Can you work these out from the drawing? Everything is in mm from the part's minimum corner. A direction names the side the tool comes from. Round coordinates to 2 decimals unless told otherwise and drop trailing zeros. Order: outer loops, then holes, each group sorted by start corner. A loop starts at its lowest first (then second) coordinate and runs counter-clockwise, first axis right, second up. Notation, with made-up numbers: (41, 75.25) -> (96, 75.25) arc R22 ccw to (96, 95.25) -> close; hole circle Ø11 at (89.25, -3). An arc over 180 degrees is marked (long way). One line per item, written item: value.
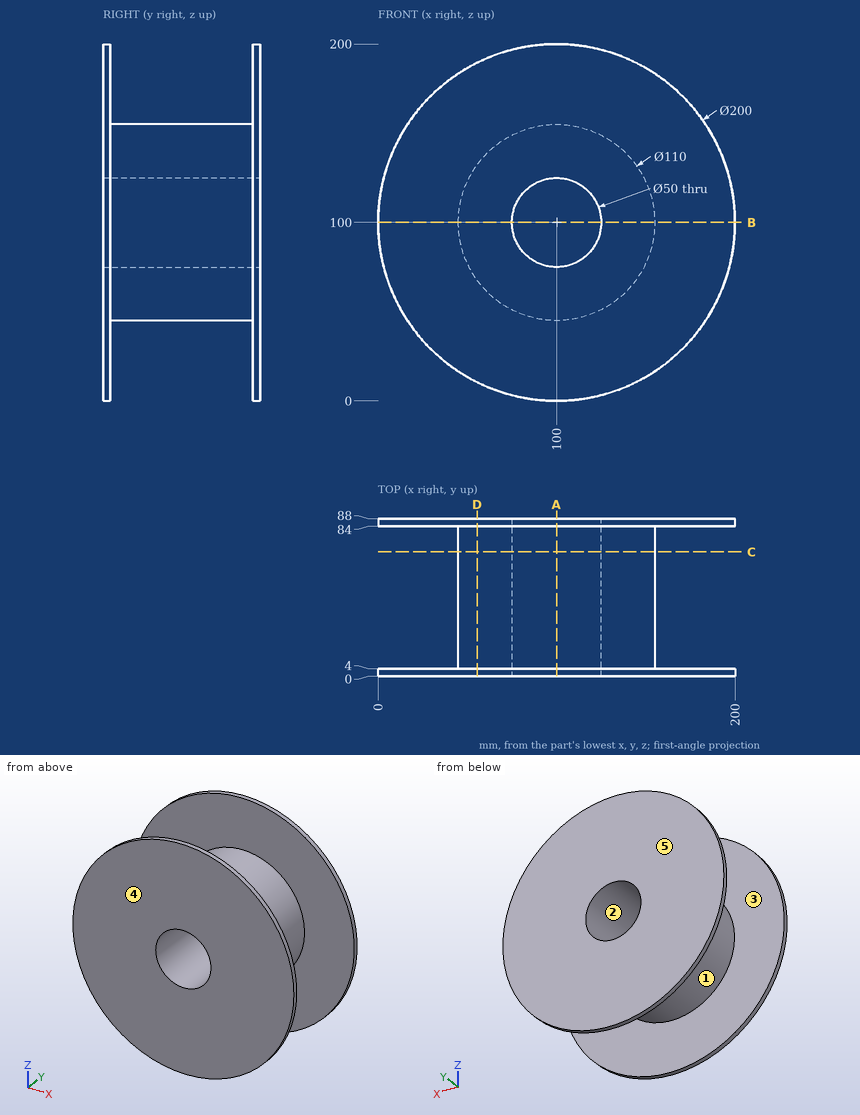
Q1. We'd pull the mould along Y, two halves only. Please class the marked faces 3, 4 and 5: released by +Y, released by -Y, zero draft, split by the parting line, or undercut.
Answers below:
face 3: undercut
face 4: released by -Y
face 5: released by +Y
Q2. Please list where these lines run through material, in increasing order: line 1 along Y through (x, z) = (160, 26); line 2 along Z through (x, y) = (100, 23); line 3 along X through (y, z) = (32, 100.5) (3 decimals).
Answers below:
line 1: 0 to 4, 84 to 88
line 2: 45 to 75, 125 to 155
line 3: 45.002 to 75.005, 124.995 to 154.998
Q3. I want a section at D-D on x = 55.5. List the corners of the cut face in (y, z) for me, plus the area to 3 significant figures.
Answers below:
outline: (0, 10.45) -> (4, 10.45) -> (4, 67.68) -> (84, 67.68) -> (84, 10.45) -> (88, 10.45) -> (88, 189.55) -> (84, 189.55) -> (84, 132.32) -> (4, 132.32) -> (4, 189.55) -> (0, 189.55) -> close
area: 6,600 mm^2
Q4. I want a section at A-A on x = 100. List the corners of the cut face in (y, z) for me, plus the area to 3 significant figures.
Answers below:
outline: (0, 0) -> (4, 0) -> (4, 45) -> (84, 45) -> (84, 0) -> (88, 0) -> (88, 75) -> (0, 75) -> close; (0, 125) -> (88, 125) -> (88, 200) -> (84, 200) -> (84, 155) -> (4, 155) -> (4, 200) -> (0, 200) -> close
area: 6,000 mm^2
Q5. On a 3-axis mill with a long thin cutter (end or side, diameter ignored), from which of +Z, -Z, +X, -X, +Y, -Y can I reach the whole of each face in a straight line? I mean the marked faces 1 and 2. Say none if no direction works.
Answers below:
face 1: none
face 2: +Y, -Y
Q6. Will these pins go through, and if not, where does the flat tip stop? pin 1 Ø8 at (x, y) = (51.5, 20) entering from +Z; pin 2 Ø5 at (y, z) = (74.5, 75.5) entering from -X; pin 3 Ø4 at (y, z) = (11, 87) entering from -X.
Answers below:
pin 1: z = 132.32
pin 2: x = 49.59
pin 3: x = 46.11
Q7. I want a section at B-B on z = 100. List the corners of the cut face in (x, y) for me, plus the area to 3 significant figures.
Answers below:
outline: (0, 0) -> (75, 0) -> (75, 88) -> (0, 88) -> (0, 84) -> (45, 84) -> (45, 4) -> (0, 4) -> close; (125, 0) -> (200, 0) -> (200, 4) -> (155, 4) -> (155, 84) -> (200, 84) -> (200, 88) -> (125, 88) -> close
area: 6,000 mm^2
Q8. I want a section at C-C on y = 69.5. List the corners of the cut face in (x, z) for me, plus the area to 3 significant figures.
Answers below:
outline: circle Ø110 at (100, 100); hole circle Ø50 at (100, 100)
area: 7,540 mm^2
